Model file for the job. Use its own axes, mm. A direction names the side the tool comes from. Round coordinates to 2 decimals unless told otherwise and drop trailing zeros. Order: outer loops, then holes, each group sorted by start corner. A loop starts at its lowest first (then second) coordinate and runs counter-clockwise, first axis right, second up. Notation, with made-up numbers: (-26, -16) -> (-6, -16) arc R9 ccw to (-6, -1) -> close; hole circle Ø6 at (67.5, 5). An arc over 180 degrees is marked (long way). Put each result on its own line as item: value. Start each with the question number.
Q1. Flat gauge pins, fed straight in: P1, Ø2, axis at y = 69, z = 1.5, coming from the +X side; P2, Ø3, axis at y = 100.5, z = 1, coming from the -X side; P3, Ø3.5, axis at x = -20.5, z = 2, coming from the +Y side. Where does each tip first touch, or does it go through?
Q2. Cut at C-C, the plane y = 60. List the corners of the cut face in (x, z), and give its area (3 significant figures).
Q3. Cut at A-A, the plane y = 7. List the corners of the cut face in (x, z), and give its area (3 significant figures).
Q4. Probe L1, parallel to Y at x = 0, z = 2.45; L2, parallel to Y at x = -20, z = -3; L3, parallel to Y at x = 7, z = 2.5. List the from-to ranges inside material, lowest first.
Q5. Cut at B-B, the plane y = 22.5. List the corners of the cut face in (x, z), and give its area (3 significant figures).
Q6. Pull direction Y, two halves, no side cores. Call faces 4 (the face through (-16, 105, -0.5)), 5 (the face through (0, 54, -3.5)): released by +Y, released by -Y, zero draft, split by the parting line, or undercut.
Q7. 3-axis set-ups, long thin cutter, end or side, ignore diameter. For faces 1 (the face through (9, 65, -0.5)), 2 (the face through (17, 38.5, 2)), 3 (the face through (19, 12, 0)): which of +Z, -Z, +X, -X, +Y, -Y reach the whole face in a straight line?
from build123d import *

# Parameters (mm, degrees)
SKETCH_1_R          = 13.25
EXTRUDE_1_DEPTH     = 3.5
SKETCH4_R           = 1.55
CUT_EXTRUDE5_DEPTH  = 5
SKETCH_2_R          = 2.1
CUT_EXTRUDE_1_DEPTH = 10
CUT_EXTRUDE_2_DEPTH = 171.144056611
FILLET_1_R          = 8
CUT_EXTRUDE_3_DEPTH = 3
SKETCH_6_R          = 25
EXTRUDE_2_DEPTH     = 7
SKETCH_7_R          = 9
SKETCH_7_R_2        = 2.05
CUT_EXTRUDE_4_DEPTH = 30
CUT_EXTRUDE_5_DEPTH = 3
SKETCH_11_R         = 3.8
SKETCH_11_R_2       = 2.05
CUT_EXTRUDE_8_DEPTH = 3
CUT_EXTRUDE_6_DEPTH = 10
CUT_EXTRUDE_7_DEPTH = 3


with BuildPart() as part:
    # 草图1 → 凸台-拉伸1 (new, symmetric)
    with BuildSketch(Plane.XY):
        with BuildLine():
            Line((-19, 0), (19, 0))
            Line((19, 0), (19, 78.751923191))
            ThreePointArc((19, 78.751923191), (0, 120), (-19, 78.751923191))
            Line((-19, 78.751923191), (-19, 0))
        make_face()
        with BuildLine():
            ThreePointArc((-8, 9), (-5, 6), (-8, 3))
            Line((-8, 3), (-14, 3))
            ThreePointArc((-14, 3), (-17, 6), (-14, 9))
            Line((-14, 9), (-8, 9))
        make_face(mode=Mode.SUBTRACT)
        with BuildLine():
            ThreePointArc((8, 3), (5, 6), (8, 9))
            Line((8, 9), (14, 9))
            ThreePointArc((14, 9), (17, 6), (14, 3))
            Line((14, 3), (8, 3))
        make_face(mode=Mode.SUBTRACT)
        with Locations((0, 95)):
            Circle(SKETCH_1_R, mode=Mode.SUBTRACT)
    extrude(amount=EXTRUDE_1_DEPTH, both=True)

    # Sketch4 → Cut-Extrude5 (cut)
    with BuildSketch(Plane(origin=(0, 0, 0), x_dir=(-1, 0, 0), z_dir=(0, -1, 0))):
        with Locations(Location((11, 0, 0), (0, 0, 180))):
            Circle(SKETCH4_R)
        with Locations((-11, 0)):
            Circle(SKETCH4_R)
    extrude(amount=-CUT_EXTRUDE5_DEPTH, mode=Mode.SUBTRACT)

    # 草图2 → 切除-拉伸1 (cut)
    with BuildSketch(Plane.XY.offset(3.5)):
        with Locations((-18.5, 95)):
            Circle(SKETCH_2_R)
        with Locations((18.5, 95)):
            Circle(SKETCH_2_R)
    extrude(amount=-CUT_EXTRUDE_1_DEPTH, mode=Mode.SUBTRACT)

    # 草图4 → 切除-拉伸2 (cut, through all)
    with BuildSketch(Plane(origin=(0, 0, -114.5), x_dir=(-1, 0, 0), z_dir=(0, 0, -1))):
        with BuildLine():
            ThreePointArc((22.386292421, 106.128967232), (0.219572962, 119.999035736), (-22.187356595, 106.520469059))
            add(Edge.make_bspline(
                [(-22.187356595, 106.520469059), (0, 122.446847778), (22.386292421, 106.128967232)],
                knots=[0, 0, 0, 1, 1, 1], degree=2))
        make_face()
    extrude(amount=-CUT_EXTRUDE_2_DEPTH, mode=Mode.SUBTRACT)

    # 圆角1
    fillet_1_edges = [part.edges().sort_by_distance(p)[0] for p in [
        (-22.386292421, 106.128967232, 0),
        (22.187356595, 106.520469059, 0),
    ]]
    fillet(fillet_1_edges, radius=FILLET_1_R)

    # 草图5 → 切除-拉伸3 (cut)
    with BuildSketch(Plane.XY.offset(-3.5)):
        Polygon((-22.238605802, 105.815360884), (0, 95), (-0.192853393, 99.54174681), (-22.228779927, 110.258538141), align=None)
        Polygon((-0.192853393, 99.54174681), (0, 95), (21.241716437, 107.661638988), (20.855269273, 112.087989547), align=None)
    extrude(amount=CUT_EXTRUDE_3_DEPTH, mode=Mode.SUBTRACT)

    # 草图6 → 凸台-拉伸2 (add)
    with BuildSketch(Plane.XY.offset(3.5)):
        with Locations((0, 40)):
            Circle(SKETCH_6_R)
    extrude(amount=-EXTRUDE_2_DEPTH)

    # 草图7 → 切除-拉伸4 (cut)
    with BuildSketch(Plane.XY.offset(3.5)):
        with Locations((0, 40)):
            Circle(SKETCH_7_R)
        with Locations((0, 60)):
            Circle(SKETCH_7_R_2)
        with Locations((17.320508076, 30)):
            Circle(SKETCH_7_R_2)
        with Locations((-17.320508076, 30)):
            Circle(SKETCH_7_R_2)
    extrude(amount=-CUT_EXTRUDE_4_DEPTH, mode=Mode.SUBTRACT)

    # 草图8 → 切除-拉伸5 (cut)
    with BuildSketch(Plane(origin=(0, 0, 3.5), x_dir=(-1, 0, 0), z_dir=(0, 0, -1))):
        Polygon((-25, 41.5), (-25, 38.5), (24.954959427, 38.5), (25.455331414, 41.5), align=None)
    extrude(amount=CUT_EXTRUDE_5_DEPTH, mode=Mode.SUBTRACT)

    # 草图11 → 切除-拉伸8 (cut)
    # profile 1 of 3: a face of its own
    with BuildSketch(Plane.XY.offset(3.5)):
        with Locations((0, 60)):
            Circle(SKETCH_11_R)
        with Locations((0, 60)):
            Circle(SKETCH_11_R_2, mode=Mode.SUBTRACT)
    # profile 2 of 3: a face of its own
    with BuildSketch(Plane.XY.offset(3.5)):
        with Locations((-17.320508076, 30)):
            Circle(SKETCH_11_R)
        with Locations((-17.320508076, 30)):
            Circle(SKETCH_11_R_2, mode=Mode.SUBTRACT)
    # profile 3 of 3: a face of its own
    with BuildSketch(Plane.XY.offset(3.5)):
        with Locations((17.320508076, 30)):
            Circle(SKETCH_11_R)
        with Locations((17.320508076, 30)):
            Circle(SKETCH_11_R_2, mode=Mode.SUBTRACT)
    extrude(amount=-CUT_EXTRUDE_8_DEPTH, mode=Mode.SUBTRACT)

    # 草图9 → 切除-拉伸6 (cut)
    with BuildSketch(Plane(origin=(0, 0, -3.5), x_dir=(-1, 0, 0), z_dir=(0, 0, -1))):
        with BuildLine():
            ThreePointArc((-10.45, 53.65506721), (-3.9, 65), (-10.45, 76.34493279))
            ThreePointArc((-10.45, 76.34493279), (-13.318653348, 75.576279442), (-12.55, 72.707626094))
            ThreePointArc((-12.55, 72.707626094), (-8.1, 65), (-12.55, 57.292373906))
            ThreePointArc((-12.55, 57.292373906), (-13.318653348, 54.423720558), (-10.45, 53.65506721))
        make_face()
    extrude(amount=-CUT_EXTRUDE_6_DEPTH, mode=Mode.SUBTRACT)

    # 草图10 → 切除-拉伸7 (cut)
    with BuildSketch(Plane(origin=(0, 0, -3.5), x_dir=(-1, 0, 0), z_dir=(0, 0, -1))):
        with BuildLine():
            ThreePointArc((-9.595, 52.17416377), (-2.19, 65), (-9.595, 77.82583623))
            ThreePointArc((-9.595, 77.82583623), (-14.799556788, 76.431279442), (-13.405, 71.226722653))
            ThreePointArc((-13.405, 71.226722653), (-9.81, 65), (-13.405, 58.773277347))
            ThreePointArc((-13.405, 58.773277347), (-14.799556788, 53.568720558), (-9.595, 52.17416377))
        make_face()
        with BuildLine():
            ThreePointArc((-12.55, 57.292373906), (-13.318653348, 54.423720558), (-10.45, 53.65506721))
            ThreePointArc((-10.45, 53.65506721), (-3.9, 65), (-10.45, 76.34493279))
            ThreePointArc((-10.45, 76.34493279), (-13.318653348, 75.576279442), (-12.55, 72.707626094))
            ThreePointArc((-12.55, 72.707626094), (-8.1, 65), (-12.55, 57.292373906))
        make_face(mode=Mode.SUBTRACT)
    extrude(amount=-CUT_EXTRUDE_7_DEPTH, mode=Mode.SUBTRACT)


solid = part.part
Ans:
1. P1: stops at x = 19
1. P2: stops at x = -24.68
1. P3: stops at y = 108.57
2. outline: (-19, -3.5) -> (-2.05, -3.5) -> (-2.05, 0.5) -> (-3.8, 0.5) -> (-3.8, 3.5) -> (-19, 3.5) -> close; (2.05, -3.5) -> (3.06, -3.5) -> (3.06, -0.5) -> (4.89, -0.5) -> (4.89, 3.5) -> (3.8, 3.5) -> (3.8, 0.5) -> (2.05, 0.5) -> close; (9.64, -0.5) -> (11.83, -0.5) -> (11.83, -3.5) -> (19, -3.5) -> (19, 3.5) -> (9.64, 3.5) -> close
2. area: 181 mm^2
3. outline: (-19, -3.5) -> (-16.83, -3.5) -> (-16.83, 3.5) -> (-19, 3.5) -> close; (-5.17, -3.5) -> (5.17, -3.5) -> (5.17, 3.5) -> (-5.17, 3.5) -> close; (16.83, -3.5) -> (19, -3.5) -> (19, 3.5) -> (16.83, 3.5) -> close
3. area: 103 mm^2
4. L1: y = 0 to 31, 49 to 56.2, 63.8 to 81.75, 108.25 to 114.39
4. L2: y = 25 to 55, 80 to 93.53, 96.47 to 104.73
4. L3: y = 0 to 3.17, 8.83 to 34.34, 45.66 to 56.54, 73.46 to 83.75, 106.25 to 113.64
5. outline: (-19, -3.5) -> (19, -3.5) -> (19, 3.5) -> (-19, 3.5) -> close
5. area: 266 mm^2
6. face 4: undercut
6. face 5: zero draft
7. face 1: -Z
7. face 2: +Z, +X, -X
7. face 3: +Z, -Z, +X, -Y
